Autodesk Inventor part; units mm, degrees
ref_plane "Work Plane1" through (0, 0, 0) normal (0, 1, 0) x (0, 0, 1)
ref_plane "Work Plane2" through (0, 40.5, 0) normal (0, 1, 0) x (0, 0, 1)
ref_plane "Work Plane3" through (0, 20.5, 0) normal (0, 1, 0) x (-1, 0, 0)
sketch "Sketch1" plane through (0, 0, 0) normal (0, 0, 1) x (1, 0, 0)
  circle A0 centre (0, 0) radius 18.6
  circle A1 centre (0, 0) radius 20.5
  dimension "d0" = 37.2
  dimension "d1" = 41
extrude "Extrusion1" add sketch "Sketch1" along normal blind 29
ref_plane "Work Plane1" through (0, 0, 0) normal (0, 1, 0) x (0, 0, 1)
ref_plane "Work Plane2" through (0, 40.5, 0) normal (0, 1, 0) x (0, 0, 1)
sketch "Sketch3" plane through (0, 0, 29) normal (0, 0, 1) x (1, 0, 0)
  circle A0 centre (0, 0) radius 20.5
  circle A1 centre (0, 0) radius 18.6
extrude "Extrusion3" add sketch "Sketch3" along normal blind 22.5
ref_plane "Work Plane3" through (0, 20.5, 0) normal (0, 1, 0) x (-1, 0, 0)
sketch "Sketch5" plane through (0, 40.5, 0) normal (0, 1, 0) x (0, 0, 1)
  line L0 (0, -20.5) -> (0, 20.5)
  line L1 (20, 20.5) -> (20, -20.5)
  point P0 (0, 0)
  dimension "d29" = 20
ref_plane "Work Plane4" through (20.5, 40.5, 20) normal (0, 0.9659, 0.2588) x (-1, 0, 0)
sketch "Sketch8" plane through (20.5, 40.5, 20) normal (0, 0.9659, 0.2588) x (-1, 0, 0)
  circle A0 centre (20.5, 3.4439) radius 12.5
  circle A1 centre (20.5, 3.4439) radius 7.9
  point P0 (20.5, -8.8363)
  dimension "d44" = 25
  dimension "d45" = 15.8
extrude "Extrusion6" add sketch "Sketch8" against normal up to surface
mirror "Mirror3" about plane through (0, 0, 0) normal (0, 0, 1) of "Extrusion1", "Extrusion6", "Extrusion3"
properties part number "JuntaEjeCadera" material "PLA"
Check sheet for the modelled part. Datum: model origin and axes. Units: mm. A direction names the side the tool comes from. Coordinates: 2 decimals unless noted, no trailing zeros. Write each loop counter-clockwise with the first axis right and the second up, starting at its lowest first coordinate (ties: lowest second). Pieces come first, ordered by that corner, then holes. Notation, with made-up numbers: (-39.5, 88) - (-13.5, 88) arc R23 cw to (-13.5, 122) - close; hole circle Ø6 at (53.5, -27). An arc over 180 degrees is marked (long way). One line per question, with ' | ' between items.
Item 1: Access from +Z, -Z, +X, -X, +Y, -Y to the whole of each face (thin tool, end or side, straight path). Record for faces 1 (the face through (0.1, 20.5, -18.1)), 2 (the face through (-9, -17, -51.5)).
Determined:
face 1: none | face 2: -Z, +X, -X, +Y, -Y
Item 2: Sectioned sample at D-D on y = -9.5. Record the boundary of the cut face in (x, z), plus the area to 3 significant figures.
Determined:
outline: (-18.17, -51.5) - (-15.99, -51.5) - (-15.99, 51.5) - (-18.17, 51.5) - close; (15.99, -51.5) - (18.17, -51.5) - (18.17, 51.5) - (15.99, 51.5) - close | area: 448 mm2
Item 3: Thickness scan on line 1 (Y direction, x = 0, z = 17); line 2 (Y direction, x = -14.5, z = 38); line 3 (X direction, y = -5, z = 46.5). Record the ranges inside material, lowest first. Write a range as [from, to].
Determined:
line 1: y = [-20.5, -18.6], [18.6, 20.5] | line 2: y = [-14.49, -11.65], [11.65, 14.49] | line 3: x = [-19.88, -17.92], [17.92, 19.88]
Item 4: Sectioned sample at A-A on y = 0. Record the boundary of the cut face in (x, z), plus the area to 3 significant figures.
Determined:
outline: (-20.5, -51.5) - (-18.6, -51.5) - (-18.6, 51.5) - (-20.5, 51.5) - close; (18.6, -51.5) - (20.5, -51.5) - (20.5, 51.5) - (18.6, 51.5) - close | area: 391 mm2
Item 5: Sectioned sample at B-B on x = 0. Record the boundary of the cut face in (y, z), plus the area to 3 significant figures.
Determined:
outline: (-20.5, -51.5) - (-18.6, -51.5) - (-18.6, 51.5) - (-20.5, 51.5) - close; (18.6, -51.5) - (20.5, -51.5) - (20.5, -31.15) - (36.37, -35.4) - (37.56, -30.96) - (20.5, -26.39) - (20.5, -10.03) - (41.65, -15.7) - (42.84, -11.25) - (20.5, -5.27) - (20.5, 5.27) - (42.84, 11.25) - (41.65, 15.7) - (20.5, 10.03) - (20.5, 26.39) - (37.56, 30.96) - (36.37, 35.4) - (20.5, 31.15) - (20.5, 51.5) - (18.6, 51.5) - close | area: 755 mm2
Item 6: Mould release check, pull along Z, two halves, no side actions. Record for faces 3 (the face through (2.71, 30.98, 8.38)), 4 (the face through (1.71, 31.09, 13.06)), 5 (the face through (9.999, 15.684, 0.721)), 6 (the face through (8.158, 39.563, -23.496)): pulls with the +Z half, pulls with the -Z half, needs draft (parallel to the pull), parting line crosses it, or undercut.
Determined:
face 3: undercut | face 4: undercut | face 5: needs draft | face 6: pulls with the -Z half
Item 7: Sectioned sample at C-C on z = 38.5. Record the boundary of the cut face in (x, y), plus the area to 3 significant figures.
Determined:
outline: circle Ø41 at (0, 0); hole circle Ø37.2 at (0, 0) | area: 233 mm2
Item 8: Gauge pin test, flat ends, axial feed: P1, Ø10, axis at y = 29, z = 27, coming from the +X side; P2, Ø5, axis at x = 9.5, z = 3.5, coming from the +Y side; P3, Ø10, axis at y = 23.5, z = 11, coming from the -X side. Record the tip position at first contact, or that the pin passes through.
Determined:
P1: stops at x = 12.43 | P2: stops at y = 19.27 | P3: stops at x = -12.2
